Source: CAD feature listing. Evaluate the final solid. Frame: model axes, mm. A direction names the side the tool comes from. Coordinates: 2 decimals unless noted, no trailing zeros. Loops run counter-clockwise (first coordinate to the right, second up) from the corner with the lowest first, then second, coordinate; pieces in that order, holes last.
Item 1: Section query B-B, the plane y = 10.5. State how many separate pieces and enclosed holes the cut face has, then the cut area to 3 significant figures.
Item 2: Reachability of faces 1 (the cylindrical face through (0, 12, 50)), 2 (the cylindrical face through (11.629, 12.325, -27.668)) from +Z, -Z, +X, -X, +Y, -Y: full face, straight path, thin tool, end or side. Return the list, or none.
Item 3: Section query A-A, the plane z = -3. Return the cut outline in (x, y), then the cut area to 3 significant figures.
Item 4: Line query: probe 1 along Z at (x, y) = (-26, 8.5); probe 2 along X at (y, z) = (19, -4.5); probe 3 along X at (y, z) = (19.25, 13). Output: solid intervals per line, ascending.
Item 5: Pin query (flat end, axial travel): pin 1 Ø10 at (x, z) = (14, 1) entering from -Y; pin 2 Ø6 at (x, y) = (46, 21.5) entering from -Z; pin 3 Ø8 at (y, z) = (16, 29.5) entering from +X; pin 4 Ø4 at (x, y) = (37.5, 10) entering from +Z. Return the tip coordinate at first contact, or that it passes through.
Item 6: Pull-direction query (X, two-part tool) for faces 3 (the flat face through (-1, 0, 1)), 4 (the cylindrical face through (-30.201, 12.325, -51.842)); classes: +X half, -X half, draft (parallel to the pull), parting line (faces both ways), or undercut.
```python
from build123d import *

# Parameters (mm, degrees)
F0_R     = 5
F2_DEPTH = 25
F3_DEPTH = 25.001


with BuildPart() as f2:
    # F0 (on Front) → F2 (new body)
    with BuildSketch(Plane.XZ):
        with BuildLine():
            ThreePointArc((-49, 9.949874), (-60, 0), (-49, -9.949874))
            ThreePointArc((-49, -9.949874), (-43.30127, -25), (-33.116844, -37.460308))
            ThreePointArc((-33.116844, -37.460308), (-31.197495, -39.073217), (-29.199711, -40.587891))
            ThreePointArc((-29.199711, -40.587891), (-23.585531, -38.505514), (-20, -43.30127))
            ThreePointArc((-20, -43.30127), (-20.139519, -44.474182), (-20.550289, -45.581637))
            ThreePointArc((-20.550289, -45.581637), (-18.239651, -46.554432), (-15.883156, -47.410182))
            ThreePointArc((-15.883156, -47.410182), (0, -50), (15.883156, -47.410182))
            ThreePointArc((15.883156, -47.410182), (18.239651, -46.554432), (20.550289, -45.581637))
            ThreePointArc((20.550289, -45.581637), (22.5, -38.971143), (29.199711, -40.587891))
            ThreePointArc((29.199711, -40.587891), (31.197495, -39.073217), (33.116844, -37.460308))
            ThreePointArc((33.116844, -37.460308), (43.30127, -25), (49, -9.949874))
            ThreePointArc((49, -9.949874), (49.437146, -7.481215), (49.75, -4.993746))
            ThreePointArc((49.75, -4.993746), (45, 0), (49.75, 4.993746))
            ThreePointArc((49.75, 4.993746), (49.437146, 7.481215), (49, 9.949874))
            ThreePointArc((49, 9.949874), (43.30127, 25), (33.116844, 37.460308))
            ThreePointArc((33.116844, 37.460308), (31.197495, 39.073217), (29.199711, 40.587891))
            ThreePointArc((29.199711, 40.587891), (22.5, 38.971143), (20.550289, 45.581637))
            ThreePointArc((20.550289, 45.581637), (18.239651, 46.554432), (15.883156, 47.410182))
            ThreePointArc((15.883156, 47.410182), (0, 50), (-15.883156, 47.410182))
            ThreePointArc((-15.883156, 47.410182), (-18.239651, 46.554432), (-20.550289, 45.581637))
            ThreePointArc((-20.550289, 45.581637), (-20.139519, 44.474182), (-20, 43.30127))
            ThreePointArc((-20, 43.30127), (-23.585531, 38.505514), (-29.199711, 40.587891))
            ThreePointArc((-29.199711, 40.587891), (-31.197495, 39.073217), (-33.116844, 37.460308))
            ThreePointArc((-33.116844, 37.460308), (-43.30127, 25), (-49, 9.949874))
        make_face()
        with Locations((-50, 0)):
            Circle(F0_R, mode=Mode.SUBTRACT)
        with BuildLine():
            ThreePointArc((-15.883156, 47.410182), (-30, 51.961524), (-33.116844, 37.460308))
            ThreePointArc((-33.116844, 37.460308), (-31.197495, 39.073217), (-29.199711, 40.587891))
            ThreePointArc((-29.199711, 40.587891), (-27.5, 47.631397), (-20.550289, 45.581637))
            ThreePointArc((-20.550289, 45.581637), (-18.239651, 46.554432), (-15.883156, 47.410182))
        make_face()
        with BuildLine():
            ThreePointArc((33.116844, 37.460308), (30, 51.961524), (15.883156, 47.410182))
            ThreePointArc((15.883156, 47.410182), (18.239651, 46.554432), (20.550289, 45.581637))
            ThreePointArc((20.550289, 45.581637), (26.172912, 48.161751), (30, 43.30127))
            ThreePointArc((30, 43.30127), (29.795756, 41.886801), (29.199711, 40.587891))
            ThreePointArc((29.199711, 40.587891), (31.197495, 39.073217), (33.116844, 37.460308))
        make_face()
        with BuildLine():
            ThreePointArc((49.75, -4.993746), (49.437146, -7.481215), (49, -9.949874))
            ThreePointArc((49, -9.949874), (60, 0), (49, 9.949874))
            ThreePointArc((49, 9.949874), (49.437146, 7.481215), (49.75, 4.993746))
            ThreePointArc((49.75, 4.993746), (53.446012, 3.622844), (55, 0))
            ThreePointArc((55, 0), (53.446012, -3.622844), (49.75, -4.993746))
        make_face()
        with BuildLine():
            ThreePointArc((20.550289, -45.581637), (18.239651, -46.554432), (15.883156, -47.410182))
            ThreePointArc((15.883156, -47.410182), (30, -51.961524), (33.116844, -37.460308))
            ThreePointArc((33.116844, -37.460308), (31.197495, -39.073217), (29.199711, -40.587891))
            ThreePointArc((29.199711, -40.587891), (29.795756, -41.886801), (30, -43.30127))
            ThreePointArc((30, -43.30127), (26.172912, -48.161751), (20.550289, -45.581637))
        make_face()
        with BuildLine():
            ThreePointArc((-29.199711, -40.587891), (-31.197495, -39.073217), (-33.116844, -37.460308))
            ThreePointArc((-33.116844, -37.460308), (-30, -51.961524), (-15.883156, -47.410182))
            ThreePointArc((-15.883156, -47.410182), (-18.239651, -46.554432), (-20.550289, -45.581637))
            ThreePointArc((-20.550289, -45.581637), (-27.5, -47.631397), (-29.199711, -40.587891))
        make_face()
    extrude(amount=-F2_DEPTH)

    # F1 (on face) → F3 (cut, through all)
    with BuildSketch(Plane.XZ):
        with BuildLine():
            ThreePointArc((-34.61205, 19.969401), (-39.616154, 5.22794), (-38.60747, -10.306999))
            ThreePointArc((-38.60747, -10.306999), (-32.51911, -13.829545), (-28.996565, -7.741185))
            ThreePointArc((-28.996565, -7.741185), (-29.754147, 3.926501), (-25.99576, 14.998238))
            ThreePointArc((-25.99576, 14.998238), (-27.818323, 21.791965), (-34.61205, 19.969401))
        make_face()
        with BuildLine():
            ThreePointArc((34.600034, 19.990214), (24.335605, 31.694626), (10.377612, 38.588549))
            ThreePointArc((10.377612, 38.588549), (4.282818, 35.077148), (7.79422, 28.982354))
            ThreePointArc((7.79422, 28.982354), (18.277524, 23.804597), (25.986735, 15.013869))
            ThreePointArc((25.986735, 15.013869), (32.781557, 13.195392), (34.600034, 19.990214))
        make_face()
        with BuildLine():
            ThreePointArc((0.012016, -39.959615), (15.280548, -36.922565), (28.229858, -28.28155))
            ThreePointArc((28.229858, -28.28155), (28.236292, -21.247603), (21.202345, -21.241169))
            ThreePointArc((21.202345, -21.241169), (11.476624, -27.731098), (0.009025, -30.012108))
            ThreePointArc((0.009025, -30.012108), (-4.963233, -34.987357), (0.012016, -39.959615))
        make_face()
    extrude(amount=-F3_DEPTH, mode=Mode.SUBTRACT)


solid = f2.part
```
Verdict:
1. separate pieces: 1
1. enclosed holes: 9
1. area: 7,310 mm2
2. face 1: +Z, +Y, -Y
2. face 2: +Y, -Y
3. outline: (-59.54, 0) - (-54, 0) - (-54, 25) - (-59.54, 25) - close; (-46, 0) - (-39.85, 0) - (-39.85, 25) - (-46, 25) - close; (-29.86, 0) - (46, 0) - (46, 25) - (-29.86, 25) - close; (54, 0) - (59.54, 0) - (59.54, 25) - (54, 25) - close
3. area: 2,330 mm2
4. probe 1: z = -53.25 to -48.2, -38.4 to 14.99, 19.98 to 38.4, 48.2 to 53.25
4. probe 2: x = -58.93 to -52.18, -47.82 to -39.71, -29.67 to 47.82, 52.18 to 58.93
4. probe 3: x = -48.28 to -37.79, -27.05 to 28.18, 32.41 to 48.28
5. pin 1: stops at y = 0
5. pin 2: stops at z = -25.51
5. pin 3: stops at x = 43.01
5. pin 4: stops at z = 35.21
6. face 3: draft
6. face 4: undercut
